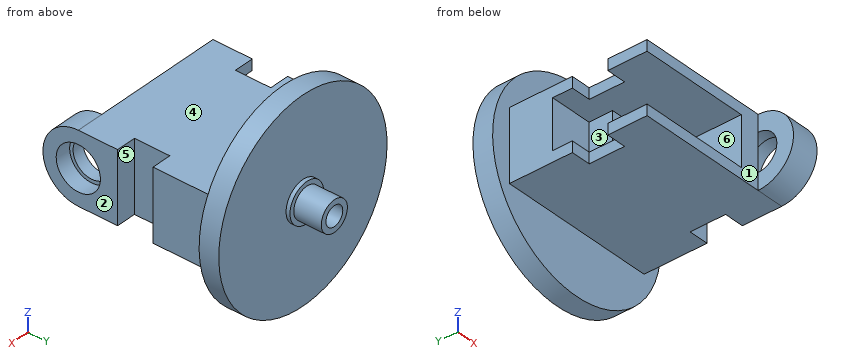
```python
from build123d import *

# Parameters (mm, degrees)
SKETCH1_R           = 25
BOSS_EXTRUDE1_DEPTH = 5
SKETCH8_R           = 4.75
BOSS_EXTRUDE3_DEPTH = 7
SKETCH9_R           = 5.625
CUT_EXTRUDE3_DEPTH  = 4
SKETCH11_W          = 33
SKETCH11_H          = 18
BOSS_EXTRUDE4_DEPTH = 35
SKETCH12_W          = 12.5
SKETCH12_H          = 18
CUT_EXTRUDE4_DEPTH  = 28
SKETCH13_W          = 12.5
SKETCH13_H          = 6
CUT_EXTRUDE6_DEPTH  = 10.79
CUT_EXTRUDE8_DEPTH  = 5
SKETCH16_R          = 5
BOSS_EXTRUDE5_DEPTH = 1
SKETCH17_R          = 3.875
BOSS_EXTRUDE6_DEPTH = 7
SKETCH18_R          = 2.5
CUT_EXTRUDE9_DEPTH  = 6
SKETCH14_R          = 3
CUT_EXTRUDE7_DEPTH  = 7


with BuildPart() as part:
    # Sketch1 → Boss-Extrude1 (new body)
    with BuildSketch(Plane(origin=(0, 0, 0), x_dir=(1, 0, 0), z_dir=(0, 1, 0))):
        with Locations(Location((0, 0, 0), (0, 0, 270))):
            Circle(SKETCH1_R)
    extrude(amount=BOSS_EXTRUDE1_DEPTH)

    # Sketch8 → Boss-Extrude3 (add)
    with BuildSketch(Plane(origin=(20, 0, 0), x_dir=(0, 0, -1), z_dir=(1, 0, 0))):
        with BuildLine():
            Line((-9, 0), (-9, -35))
            ThreePointArc((-9, -35), (0, -44), (9, -35))
            Line((9, -35), (9, 0))
            Line((9, 0), (-9, 0))
        make_face()
        with Locations((0, -35)):
            Circle(SKETCH8_R, mode=Mode.SUBTRACT)
    extrude(amount=-BOSS_EXTRUDE3_DEPTH)

    # Sketch9 → Cut-Extrude3 (cut)
    with BuildSketch(Plane.ZY.offset(-20)):
        with Locations((0, -35)):
            Circle(SKETCH9_R)
    extrude(amount=CUT_EXTRUDE3_DEPTH, mode=Mode.SUBTRACT)

    # Sketch11 → Boss-Extrude4 (add)
    with BuildSketch(Plane(origin=(0, 0, 0), x_dir=(-1, 0, 0), z_dir=(0, -1, 0))):
        with Locations((3.5, 0)):
            Rectangle(SKETCH11_W, SKETCH11_H)
    extrude(amount=BOSS_EXTRUDE4_DEPTH)

    # Sketch12 → Cut-Extrude4 (cut)
    with BuildSketch(Plane.ZY.offset(20)):
        with Locations((0, -26)):
            Rectangle(SKETCH12_W, SKETCH12_H)
    extrude(amount=-CUT_EXTRUDE4_DEPTH, mode=Mode.SUBTRACT)

    # Sketch13 → Cut-Extrude6 (cut)
    with BuildSketch(Plane.ZY.offset(20)):
        with Locations((0, -14)):
            Rectangle(SKETCH13_W, SKETCH13_H)
    extrude(amount=-CUT_EXTRUDE6_DEPTH, mode=Mode.SUBTRACT)

    # Sketch15 → Cut-Extrude8 (cut)
    with BuildSketch(Plane.ZY.offset(20)):
        Polygon((-6.25, -25), (-9, -25), (-9, -16), (-6.25, -16), (9, -16), (9, -25), align=None)
    cut_extrude8 = extrude(amount=-CUT_EXTRUDE8_DEPTH, mode=Mode.SUBTRACT)

    # Mirror1: Cut-Extrude8 across plane
    add(cut_extrude8.mirror(Plane.ZY), mode=Mode.SUBTRACT)

    # Sketch16 → Boss-Extrude5 (add)
    with BuildSketch(Plane(origin=(0, 5, 0), x_dir=(1, 0, 0), z_dir=(0, 1, 0))):
        with Locations(Location((0, 0, 0), (0, 0, 270))):
            Circle(SKETCH16_R)
    extrude(amount=BOSS_EXTRUDE5_DEPTH)

    # Sketch17 → Boss-Extrude6 (add)
    with BuildSketch(Plane(origin=(0, 6, 0), x_dir=(1, 0, 0), z_dir=(0, 1, 0))):
        with Locations(Location((0, 0, 0), (0, 0, 270))):
            Circle(SKETCH17_R)
    extrude(amount=BOSS_EXTRUDE6_DEPTH)

    # Sketch18 → Cut-Extrude9 (cut)
    with BuildSketch(Plane(origin=(0, 13, 0), x_dir=(1, 0, 0), z_dir=(0, 1, 0))):
        with Locations(Location((0, 0, 0), (0, 0, 270))):
            Circle(SKETCH18_R)
    extrude(amount=-CUT_EXTRUDE9_DEPTH, mode=Mode.SUBTRACT)

    # Sketch14 → Cut-Extrude7 (cut)
    with BuildSketch(Plane(origin=(0, 5, 0), x_dir=(1, 0, 0), z_dir=(0, 1, 0))):
        with Locations(Location((0, 0, 0), (0, 0, 270))):
            Circle(SKETCH14_R)
    extrude(amount=-CUT_EXTRUDE7_DEPTH, mode=Mode.SUBTRACT)


solid = part.part
```
Verification items for the finished model (mm, model axes). Face numbers are marked on the shaded views. A direction names the side the tool comes from. Give positions to 0.01 mm unless a question says otherwise; leave off trailing zeros. Order: outer loops, then holes, each group sorted by start corner. A loop starts at its lowest first (then second) coordinate and runs counter-clockwise, first axis right, second up. Notation, with made-up numbers: M 49,56 L 95,56 A24 ccw 95,87 Z; hole C -32.5,-25 d4. An arc over 180 degrees is marked long. Answer in a Markdown table with one row per item. Add a question column.
Item 1: Scan lines: probe 1 along Z at (x, y) = (-16, -15.5); probe 2 along X at (y, z) = (11.6, 0) (3 decimals); probe 3 along X at (y, z) = (-0.5, 0). Record each from-to range of solid material in increasing order. Write a range as from..to.
Item 2: Gauge pin test, flat ends, axial feed: pin 1 (1.5 mm diameter, centred on x = 18, y = -30.5, fed in from -Z); pin 2 (2 mm diameter, centred on x = -17.5, z = 7.5, fed in from +Y); pin 3 (3 mm diameter, centred on x = -16.5, z = 7.5, fed in from -Y). Record the tip position at first contact, or that the pin passes through.
Item 3: Section check A-A, the plane z = 0. State how many separate pieces and enclosed holes the cut face has, and give its area (3 significant figures).
Item 4: Section check B-B, the plane y = 8.5. Enter the section's corners in (x, z) (3 decimals).
Item 5: Section check C-C, the plane x = -12.5. Enter the section's corners in (y, z), and give its area (3 significant figures).
Item 6: Tool access check on the marked faces 1, 2 and 3. Record the directions out of +Z, -Z, +X, -X, +Y, -Y that give a thin tool (end or side, any length) a straight path to the whole face; none if there is none.
Item 7: Mould release check, pull along Z, two halves, no side actions. Record for the marked faces 4, 5 and 6: released by +Z, released by -Z, zero draft, split by the parting line, or undercut.
Item 8: Section check D-D, the plane y = -28.5. Enter the section's corners in (x, z), and give its area (3 significant figures).
Filled sheet:
| question | item | result |
|---|---|---|
| 1 | probe 1 | z = -9..-6.25, 6.25..9 |
| 1 | probe 2 | x = -3.875..-2.5, 2.5..3.875 |
| 1 | probe 3 | x = -20..-3, 3..20 |
| 2 | pin 1 | stops at z = -9 |
| 2 | pin 2 | stops at y = 5 |
| 2 | pin 3 | stops at y = -35 |
| 3 | separate pieces | 2 |
| 3 | enclosed holes | 1 |
| 3 | area | 1,020 mm^2 |
| 4 | outline | C 0,0 d7.75; hole C 0,0 d5 |
| 5 | outline | M -35,-9 L 0,-9 L 0,-21.65 L 5,-21.65 L 5,21.65 L 0,21.65 L 0,9 L -35,9 L -35,6.25 L -11,6.25 L -11,-6.25 L -35,-6.25 Z |
| 5 | area | 547 mm^2 |
| 6 | face 1 | +Z, -Z, -X, -Y |
| 6 | face 2 | +Z, -Z, +X, -Y |
| 6 | face 3 | -X, -Y |
| 7 | face 4 | released by +Z |
| 7 | face 5 | zero draft |
| 7 | face 6 | undercut |
| 8 | outline | M -20,-9 L 20,-9 L 20,9 L -20,9 L -20,6.25 L 8,6.25 L 8,-6.25 L -20,-6.25 Z |
| 8 | area | 370 mm^2 |
